from build123d import *

# Parameters (mm, degrees)
BOSS_EXTRUDE1_DEPTH                                 = 1492.25
CSK_FOR_1_4_FLAT_HEAD_SOCKET_CAP_SCREW1_D           = 7.14248
CSK_FOR_1_4_FLAT_HEAD_SOCKET_CAP_SCREW1_CSINK_D     = 13.4874
CSK_FOR_1_4_FLAT_HEAD_SOCKET_CAP_SCREW1_CSINK_ANGLE = 82
SKETCH4_R                                           = 22.225
CUT_EXTRUDE1_DEPTH                                  = 67.312434508
CUT_EXTRUDE2_DEPTH                                  = 67.312434508
FILLET1_R                                           = 6.35


with BuildPart() as part:
    # Sketch1 → Boss-Extrude1 (new body)
    with BuildSketch(Plane.XY):
        Polygon((22.225, 55.50367642), (229.367540407, 0), (278.436572382, 0), (25.512001873, 67.770934414), align=None)
    extrude(amount=BOSS_EXTRUDE1_DEPTH)

    # CSK for 1/4 Flat Head Socket Cap Screw1 (through all)
    with Locations(Plane(origin=(18.651713678, 69.609143096, 0), x_dir=(0.965925826, -0.258819045, 0), z_dir=(0.258819045, 0.965925826, 0))):
        with Locations((44.668892959, -1251.74375), (70.068892959, -1251.74375), (44.668892959, -770.73125), (70.068892959, -770.73125), (44.668892959, -1473.2), (70.068892959, -1473.2), (44.668892959, -342.9), (70.068892959, -342.9)):
            CounterSinkHole(CSK_FOR_1_4_FLAT_HEAD_SOCKET_CAP_SCREW1_D / 2, CSK_FOR_1_4_FLAT_HEAD_SOCKET_CAP_SCREW1_CSINK_D / 2, counter_sink_angle=CSK_FOR_1_4_FLAT_HEAD_SOCKET_CAP_SCREW1_CSINK_ANGLE)

    # Sketch4 → Cut-Extrude1 (cut, through all)
    with BuildSketch(Plane(origin=(18.651713678, 69.609143096, 0), x_dir=(0.965925826, -0.258819045, 0), z_dir=(0.258819045, 0.965925826, 0))):
        with Locations((7.102292959, -770.73125)):
            Circle(SKETCH4_R)
        with Locations((7.102292959, -1251.74375)):
            Circle(SKETCH4_R)
    extrude(amount=-CUT_EXTRUDE1_DEPTH, mode=Mode.SUBTRACT)

    # Sketch5 → Cut-Extrude2 (cut, through all)
    with BuildSketch(Plane(origin=(18.651713678, 69.609143096, 0), x_dir=(0.965925826, -0.258819045, 0), z_dir=(0.258819045, 0.965925826, 0))):
        Polygon((7.102292959, -317.5), (7.102292959, 0), (268.949076248, 0), (32.502292959, -240.609994719), (32.502292959, -317.5), align=None)
    extrude(amount=-CUT_EXTRUDE2_DEPTH, mode=Mode.SUBTRACT)

    # Fillet1
    fillet1_edges = [part.edges().sort_by_distance(p)[0] for p in [
        (48.403016924, 55.063301672, 317.5),
    ]]
    fillet(fillet1_edges, radius=FILLET1_R)


solid = part.part
Can you work these out from the model? Positions are in its coordinate system, mm. Round coordinates to 2 decimals unless told otherwise and drop trailing zeros. Loops run counter-clockwise (first coordinate to the right, second up) from the corner with the lowest first, then second, coordinate; pieces in that order, holes last. Notation, with made-up numbers: (84, 41) - (99, 41) arc R33 cw to (99, 74) - close; hole circle Ø4 at (-9, 20.5). An arc over 180 degrees is marked (long way). Use CSV: the item, a comma, the result in double quotes. Start each with the question number.
1) We'd pull the mould along Z, two halves only. Please class faces 1 (the flat face through (140, 32, 1492.25)), 2 (the cylindrical face through (45.354, 55.972, 1252.232)), 3 (the flat face through (254, 0, 736)): released by +Z, released by -Z, zero draft, split by the parting line, or undercut.
2) For pin 1 Ø2 at (x, z) = (128.5, 286) entering from +Y; pin 2 Ø6 at (x, z) = (80.5, 1119) entering from -Y; pin 3 Ø5 at (x, y) = (33, 59.5) entering from -Z, each with a flat end and sliding along its axis, tell me the tip position at first contact or that it passes through.
3) If we section it at B-B on y = 19: Write out the boundary of the cut face in (x, z).
4) If we section it at A-A on z = 292.5: Write out the boundary of the cut face in (x, y).
5) Please list where these lines run through material, in increasing order: probe 1 along Y at (x, z) = (75, 760); probe 2 along Y at (x, z) = (249.5, 517). Write a range as [from, to].
Geometry results:
1,face 1,"released by +Z"
1,face 2,"undercut"
1,face 3,"zero draft"
2,pin 1,"stops at y = 40.44"
2,pin 2,"stops at y = 39.09"
2,pin 3,"stops at z = 317.5"
3,outline,"(158.46, 122.93) - (207.53, 74.7) - (207.53, 1492.25) - (158.46, 1492.25) - close"
4,outline,"(46.76, 48.93) - (229.37, 0) - (278.44, 0) - (50.05, 61.2) - close"
5,probe 1,"y = [41.36, 54.51]"
5,probe 2,"y = [0, 7.75]"
